Read the model definition and answer for the solid it produces. Units are mm, in the model's axes. A direction names the side the tool comes from. Coordinates: 2 decimals unless noted, no trailing zeros. Loops run counter-clockwise (first coordinate to the right, second up) from the corner with the lowest first, then second, coordinate; pieces in that order, holes last. Notation, with made-up numbers: M 72,37.25 L 113,37.25 A17 cw 113,55.25 Z; hole C 80,0 d8. An arc over 180 degrees is marked long. One line per item, written item: value. Start each with the question number.
```python
from build123d import *

# Parameters (mm, degrees)
BOSS_EXTRUDE1_DEPTH = 3
CUT_EXTRUDE1_START  = -2.5
CUT_EXTRUDE1_DEPTH  = 2.5
FILLET1_R           = 0.5
SKETCH3_R           = 0.4
BOSS_EXTRUDE2_DEPTH = 2
FILLET2_R           = 0.1


with BuildPart() as part:
    # Sketch1 → Boss-Extrude1 (new body)
    with BuildSketch(Plane(origin=(0, 0, 0), x_dir=(1, 0, 0), z_dir=(0, 1, 0))):
        with BuildLine():
            Line((-3.5, 2), (3.5, 2))
            ThreePointArc((3.5, 2), (5.5, 0), (3.5, -2))
            Line((3.5, -2), (-3.5, -2))
            ThreePointArc((-3.5, -2), (-5.5, 0), (-3.5, 2))
        make_face()
    extrude(amount=BOSS_EXTRUDE1_DEPTH)

    # Sketch2 → Cut-Extrude1 (cut)
    with BuildSketch(Plane(origin=(0, 3, 0), x_dir=(1, 0, 0), z_dir=(0, 1, 0)).offset(CUT_EXTRUDE1_START)):
        with BuildLine():
            Line((-3.5, -2), (3.5, -2))
            ThreePointArc((3.5, -2), (5.5, 0), (3.5, 2))
            Line((3.5, 2), (-3.5, 2))
            ThreePointArc((-3.5, 2), (-5.5, 0), (-3.5, -2))
        make_face()
        with BuildLine():
            Line((-3.5, -1.75), (3.5, -1.75))
            ThreePointArc((3.5, -1.75), (5.25, 0), (3.5, 1.75))
            Line((3.5, 1.75), (-3.5, 1.75))
            ThreePointArc((-3.5, 1.75), (-5.25, 0), (-3.5, -1.75))
        make_face(mode=Mode.SUBTRACT)
    extrude(amount=CUT_EXTRUDE1_DEPTH, mode=Mode.SUBTRACT)

    # Fillet1
    fillet1_edges = [part.edges().sort_by_distance(p)[0] for p in [
        (-5.25, 3, 0),
        (0, 3, -1.75),
        (5.25, 3, 0),
        (0, 3, 1.75),
    ]]
    fillet(fillet1_edges, radius=FILLET1_R)

    # Sketch3 → Boss-Extrude2 (add)
    with BuildSketch(Plane.XZ):
        with Locations(Location((-2.54, 0, 0), (0, 0, 90))):
            Circle(SKETCH3_R)
        with Locations(Location((2.54, 0, 0), (0, 0, 90))):
            Circle(SKETCH3_R)
    extrude(amount=BOSS_EXTRUDE2_DEPTH)

    # Fillet2
    fillet2_edges = [part.edges().sort_by_distance(p)[0] for p in [
        (0, 0.5, -1.75),
        (-5.25, 0.5, 0),
        (0, 0.5, 1.75),
        (5.25, 0.5, 0),
    ]]
    fillet(fillet2_edges, radius=FILLET2_R)


solid = part.part
```
1) Section C-C (z = 0) is taken. Determine the outline of the cut face in (x, y).
2) Section A-A (x = 2) is taken. Determine the outline of the cut face in (y, z), then the cut area to 3 significant figures.
3) A tool of negligible diameter and unlimited length cuts with its end or side. For faces 1 (the face through (5.25, 1.54, 0.04)), 2 (the face through (0, 2, -1.75)), 3 (the face through (-5.25, 1.54, -0.04)), from which of +Z, -Z, +X, -X, +Y, -Y can it reach the whole face along a straight path? Write none if from no direction.
4) Consider line 1 along X through (y, z) = (-0.6, 0); line 2 along Y through (x, z) = (3.25, 0.35); line 3 along Z through (x, y) = (3.25, 1.5). Determine where each line is inside the solid, lowest interval first.
5) Section B-B (y = -0.3) is taken. Determine the outline of the cut face in (x, z), then the cut area to 3 significant figures.
6) Section D-D (x = -2.54) is taken. Determine the outline of the cut face in (y, z).
7) Flat-ended cylindrical pins translate along their axes: pin 1 (0.6 mm diameter, centred on x = -1, y = 1.5, fed in from -Z); pin 2 (1.5 mm diameter, centred on x = 1.5, y = 1.5, fed in from +Z); pin 3 (1 mm diameter, centred on y = 2.5, z = 0.5, fed in from -X). Find the tip coordinate at first contact, or state that the pin passes through.
Results found:
1. outline: M -5.5,0 L -2.94,0 L -2.94,-2 L -2.14,-2 L -2.14,0 L 2.14,0 L 2.14,-2 L 2.94,-2 L 2.94,0 L 5.5,0 L 5.5,0.5 L 5.35,0.5 A0.1 cw 5.25,0.6 L 5.25,2.5 A0.5 ccw 4.75,3 L -4.75,3 A0.5 ccw -5.25,2.5 L -5.25,0.6 A0.1 cw -5.35,0.5 L -5.5,0.5 Z
2. outline: M 0,-2 L 0.5,-2 L 0.5,-1.85 A0.1 cw 0.6,-1.75 L 2.5,-1.75 A0.5 ccw 3,-1.25 L 3,1.25 A0.5 ccw 2.5,1.75 L 0.6,1.75 A0.1 cw 0.5,1.85 L 0.5,2 L 0,2 Z
2. area: 10.6 mm²
3. face 1: +X, +Y
3. face 2: -Z, +X, -X, +Y
3. face 3: -X, +Y
4. line 1: x = -2.94 to -2.14, 2.14 to 2.94
4. line 2: y = 0 to 3
4. line 3: z = -1.75 to 1.75
5. outline: C -2.54,0 d0.8; C 2.54,0 d0.8
5. area: 1.01 mm²
6. outline: M -2,-0.4 L 0,-0.4 L 0,-2 L 0.5,-2 L 0.5,-1.85 A0.1 cw 0.6,-1.75 L 2.5,-1.75 A0.5 ccw 3,-1.25 L 3,1.25 A0.5 ccw 2.5,1.75 L 0.6,1.75 A0.1 cw 0.5,1.85 L 0.5,2 L 0,2 L 0,0.4 L -2,0.4 Z
7. pin 1: stops at z = -1.75
7. pin 2: stops at z = 1.75
7. pin 3: stops at x = -5.25
